Can you work these out from the model? Positions are in its coordinate system, mm. Face numbers are marked on the shaded views. A direction names the side the tool comes from. Give positions to 0.01 mm unless a question says otherwise; leave off trailing zeros. Write each loop counter-clockwise with the first axis right and the second up, starting at its lowest first coordinate (ties: lowest second). Pieces come first, ordered by that corner, then holes. Notation, with made-up numbers: M 48,69 L 60,69 A15 cw 60,97 Z; hole C -32,-22.75 d10. An arc over 180 degrees is marked long. Write each question's results on one line, items separated by ' | '.
from build123d import *

# Parameters (mm, degrees)
SKETCH1_R           = 2.5
SKETCH1_R_2         = 2.25
SKETCH1_W           = 8
SKETCH1_H           = 5
BOSS_EXTRUDE1_DEPTH = 2.5
EXTRUDE_START       = 3
SKETCH_2_R          = 8
SKETCH_2_R_2        = 2
EXTRUDE_1_DEPTH     = 3


with BuildPart() as part:
    # Sketch1 → Boss-Extrude1 (new, symmetric)
    with BuildSketch(Plane.XY):
        with BuildLine():
            Line((-27.5, 0), (27.5, 0))
            ThreePointArc((27.5, 0), (36.5, 9), (27.5, 18))
            Line((27.5, 18), (11.1, 18))
            ThreePointArc((11.1, 18), (4.028932188, 20.928932188), (1.1, 28))
            Line((1.1, 28), (1.1, 33))
            ThreePointArc((1.1, 33), (-6.9, 41), (-14.9, 33))
            Line((-14.9, 33), (-14.9, 22))
            ThreePointArc((-14.9, 22), (-17.828932188, 14.928932188), (-24.9, 12))
            Line((-24.9, 12), (-27.5, 12))
            ThreePointArc((-27.5, 12), (-33.5, 6), (-27.5, 0))
        make_face()
        with Locations((27.5, 9)):
            Circle(SKETCH1_R, mode=Mode.SUBTRACT)
        with Locations((-27.5, 6)):
            Circle(SKETCH1_R_2, mode=Mode.SUBTRACT)
        with Locations((-6.9, 33)):
            Circle(SKETCH1_R_2, mode=Mode.SUBTRACT)
        with Locations((-11.5, 6)):
            Rectangle(SKETCH1_W, SKETCH1_H, mode=Mode.SUBTRACT)
        with Locations((6.5, 6)):
            Rectangle(SKETCH1_W, SKETCH1_H, mode=Mode.SUBTRACT)
    extrude(amount=BOSS_EXTRUDE1_DEPTH, both=True)

    # 草图2 → 凸台-拉伸1 (add)
    with BuildSketch(Plane.XY.offset(2.5).offset(EXTRUDE_START)):
        with Locations((-6.9, 33)):
            Circle(SKETCH_2_R)
        with Locations((-6.9, 33)):
            Circle(SKETCH_2_R_2, mode=Mode.SUBTRACT)
    extrude(amount=-EXTRUDE_1_DEPTH)


solid = part.part
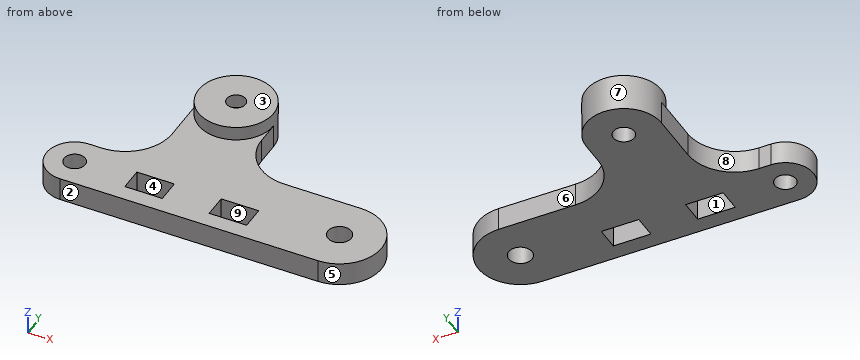
Item 1: For the marked faces 5, 6, 7, 8 and 9, which set-ups out of +Z, -Z, +X, -X, +Y, -Y let a thin tool reach every point of the face, with its end or its side?
Geometry says:
face 5: +Z, -Z, +X | face 6: +Z, -Z, +X, +Y | face 7: +Z | face 8: +Z, -Z, -X, +Y | face 9: +Z, -Z
Item 2: I want a section at C-C, the plane x = 8. Please give me the cut outline in (y, z), and give its area (3 significant figures).
Geometry says:
outline: M 0,-2.5 L 3.5,-2.5 L 3.5,2.5 L 0,2.5 Z; M 8.5,-2.5 L 18.49,-2.5 L 18.49,2.5 L 8.5,2.5 Z | area: 67.5 mm2
Item 3: I'm going to push flat-ended pins straight in: pin 1 (4 mm diameter, centred on y = 27.5, z = -0.5, fed in from -X); pin 2 (3 mm diameter, centred on x = -25.5, z = 1, fed in from +Y); pin 3 (4 mm diameter, centred on x = 27.5, y = 9, fed in from +Z); pin 4 (10 mm diameter, centred on x = 26.5, y = 6, fed in from +Z). Where does each tip first touch, or does it pass through?
Geometry says:
pin 1: stops at x = -14.9 | pin 2: stops at y = 12.04 | pin 3: passes through | pin 4: stops at z = 2.5
Item 4: I want a section at A-A, the plane x = 28.5. Please give me the cut outline in (y, z), and give its area (3 significant figures).
Geometry says:
outline: M 0.06,-2.5 L 6.71,-2.5 L 6.71,2.5 L 0.06,2.5 Z; M 11.29,-2.5 L 17.94,-2.5 L 17.94,2.5 L 11.29,2.5 Z | area: 66.5 mm2
Item 5: I want a section at B-B, the plane z = 1. Please give me the cut outline in (x, y).
Geometry says:
outline: M -27.5,0 L 27.5,0 A9 ccw 27.5,18 L 11.1,18 A10 cw 1.1,28 L 1.1,33 A8 ccw -14.9,33 L -14.9,22 A10 cw -24.9,12 L -27.5,12 A6 ccw Z; hole C -27.5,6 d4.5; hole M -15.5,3.5 L -7.5,3.5 L -7.5,8.5 L -15.5,8.5 Z; hole C -6.9,33 d4.5; hole M 2.5,3.5 L 10.5,3.5 L 10.5,8.5 L 2.5,8.5 Z; hole C 27.5,9 d5
Item 6: If I drill on line 1 (Y direction, x = -27.5, z = -1.4); line 2 (Y direction, x = 27.5, z = 2.25); line 3 (X direction, y = 7, z = 0.75), over which ranges is the centre line in solid material (lowest first)? Write a range as from..to.
Geometry says:
line 1: y = 0..3.75, 8.25..12 | line 2: y = 0..6.5, 11.5..18 | line 3: x = -33.42..-29.52, -25.48..-15.5, -7.5..2.5, 10.5..26, 29..36.27
Item 7: Thinking about a two-plate mould opening in Y: for the marked faces 1, 2, 3 and 4, which applies, +Y half, -Y half, draft (parallel to the pull), parting line (faces both ways), or undercut?
Geometry says:
face 1: undercut | face 2: -Y half | face 3: draft | face 4: undercut
Item 8: I want a section at D-D, the plane z = 4. Please give me the cut outline in (x, y).
Geometry says:
outline: C -6.9,33 d16; hole C -6.9,33 d4
